Here's how the part is built. I have some questions about the finished solid (model axes, mm). A direction names the side the tool comes from. Round coordinates to 2 decimals unless told otherwise and drop trailing zeros. Loops run counter-clockwise (first coordinate to the right, second up) from the corner with the lowest first, then second, coordinate; pieces in that order, holes last. Notation, with made-up numbers: (70, -8.5) -> (98, -8.5) arc R35 ccw to (98, 28.5) -> close; hole circle Ø3 at (15.25, 10). An arc over 180 degrees is marked (long way). Use one line per item in the form item = value. Start each with the question number.
Item 1: For faces 1 (the face through (2, -12, 4)), 2 (the face through (0, -12, 3)), 3 (the face through (9, 14.2, 4)), 4 (the face through (1.43, 1.4, 4.54)), which set-ups out of +Z, -Z, +X, -X, +Y, -Y let a thin tool reach every point of the face, with its end or its side?
Item 2: Thinking about a two-plate mould opening in Y: for faces 5 (the face through (8, 4, 2)), 6 (the face through (-5, 1, 7)), 7 (the face through (28, 0, 3)), which applies, released by +Y, released by -Y, zero draft, split by the parting line, or undercut?
Item 3: If we section it at D-D (y = 10.5): Write out the boundary of the cut face in (x, z), then the cut area to 3 significant figures.
Item 4: I'm going to push flat-ended pins straight in: pin 1 Ø1.5 at (x, y) = (5.5, 9) entering from -Z; pin 2 Ø2.5 at (x, z) = (19, 5) entering from -Y; pin 3 Ø3.5 at (y, z) = (-11, 3.5) entering from +X; pin 4 Ø2.5 at (y, z) = (-14, 5.5) entering from -X. Where does each tip first touch, or does it pass through?
Item 5: If I drill on L1, parallel to Y at x = 21, z = 5.25; L2, parallel to Z at x = 1, y = 3, over which ranges is the centre line in solid material (lowest first)? Write a range as [from, to].
Item 6: If we section it at A-A (z = 3.25): Write out the boundary of the cut face in (x, y).
Item 7: If we section it at B-B (y = -12.5): Write out the boundary of the cut face in (x, z).
```python
from build123d import *

# Parameters (mm, degrees)
PAD_DEPTH   = 7
THICKNESS_T = -2


with BuildPart() as part:
    # Sketch001 → Pad (new body)
    with BuildSketch(Plane.XY):
        Polygon((0, 0), (0, -23.8), (16.2, -23.8), (16.2, 0), (40, 0), (40, 16.2), (-23.8, 16.2), (-23.8, 0), align=None)
    extrude(amount=PAD_DEPTH)

    # Thickness
    thickness_openings = [part.faces().sort_by_distance(p)[0] for p in [
        (8.1, 2.66621, 7),
        (8.1, -23.8, 3.5),
        (40, 8.1, 3.5),
        (-23.8, 8.1, 3.5),
    ]]
    offset(amount=THICKNESS_T, openings=thickness_openings)


solid = part.part
```
Values found:
q1.face_1 = +Z, -Y
q1.face_2 = +Z, -Z, -X, -Y
q1.face_3 = +Z, +X, -X
q1.face_4 = +Z
q2.face_5 = undercut
q2.face_6 = zero draft
q2.face_7 = released by -Y
q3.outline = (-23.8, 0) -> (40, 0) -> (40, 2) -> (-23.8, 2) -> close
q3.area = 128 mm2
q4.pin_1 = 0
q4.pin_2 = 0
q4.pin_3 = 16.2
q4.pin_4 = 0
q5.L1 = [0, 2], [14.2, 16.2]
q5.L2 = [0, 2]
q6.outline = (-23.8, 0) -> (0, 0) -> (0, -23.8) -> (2, -23.8) -> (2, 0) arc R2 ccw to (0, 2) -> (-23.8, 2) -> close; (-23.8, 14.2) -> (40, 14.2) -> (40, 16.2) -> (-23.8, 16.2) -> close; (14.2, -23.8) -> (16.2, -23.8) -> (16.2, 0) -> (40, 0) -> (40, 2) -> (16.2, 2) arc R2 ccw to (14.2, 0) -> close
q7.outline = (0, 0) -> (16.2, 0) -> (16.2, 7) -> (14.2, 7) -> (14.2, 2) -> (2, 2) -> (2, 7) -> (0, 7) -> close
